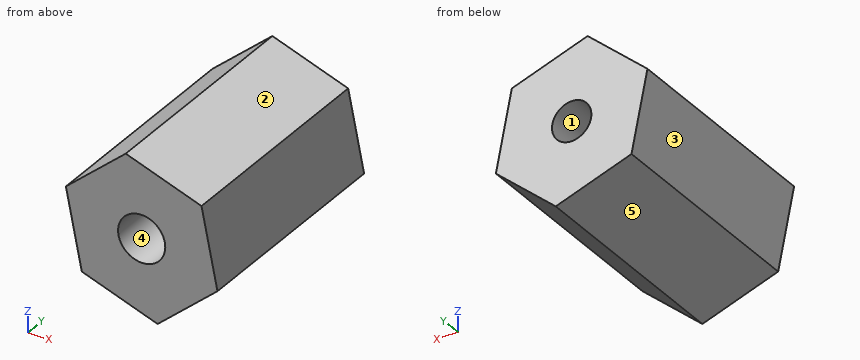
```python
from build123d import *

# Parameters (mm, degrees)
BOSS_EXTRUDE1_DEPTH       = 12.7
F_4_40_TAPPED_HOLE1_D     = 2.2606
F_4_40_TAPPED_HOLE1_DEPTH = 3.571875
F_4_40_TAPPED_HOLE1_TIP   = 0.679152758
F_6_32_TAPPED_HOLE1_D     = 2.7051
F_6_32_TAPPED_HOLE1_DEPTH = 3.556
F_6_32_TAPPED_HOLE1_TIP   = 0.81269403


with BuildPart() as part:
    # Sketch1 → Boss-Extrude1 (new body)
    with BuildSketch(Plane(origin=(0, 0, 0), x_dir=(1, 0, 0), z_dir=(0, 1, 0))):
        Polygon((3.431522356, -3.037425951), (4.346249213, 1.453072558), (0.914726858, 4.490498509), (-3.431522356, 3.037425951), (-4.346249213, -1.453072558), (-0.914726858, -4.490498509), align=None)
    extrude(amount=BOSS_EXTRUDE1_DEPTH)

    # #4-40 Tapped Hole1
    with Locations(Plane(origin=(0, 12.7, 0), x_dir=(1, 0, 0), z_dir=(0, 1, 0))):
        with Locations((0, 0)):
            Hole(F_4_40_TAPPED_HOLE1_D / 2, depth=F_4_40_TAPPED_HOLE1_DEPTH)
            with Locations((0, 0, -(F_4_40_TAPPED_HOLE1_DEPTH + F_4_40_TAPPED_HOLE1_TIP / 2))):  # 118° drill point
                Cone(0, F_4_40_TAPPED_HOLE1_D / 2, F_4_40_TAPPED_HOLE1_TIP, mode=Mode.SUBTRACT)

    # #6-32 Tapped Hole1
    with Locations(Plane(origin=(0, 0, 0), x_dir=(-1, 0, 0), z_dir=(0, -1, 0))):
        with Locations((0, 0)):
            Hole(F_6_32_TAPPED_HOLE1_D / 2, depth=F_6_32_TAPPED_HOLE1_DEPTH)
            with Locations((0, 0, -(F_6_32_TAPPED_HOLE1_DEPTH + F_6_32_TAPPED_HOLE1_TIP / 2))):  # 118° drill point
                Cone(0, F_6_32_TAPPED_HOLE1_D / 2, F_6_32_TAPPED_HOLE1_TIP, mode=Mode.SUBTRACT)


solid = part.part
```
Read the model definition and answer for the solid it produces. Units are mm, in the model's axes. Face numbers are marked on the shaded views. A direction names the side the tool comes from. Give positions to 0.01 mm unless a question says otherwise; leave off trailing zeros. Write each loop counter-clockwise with the first axis right and the second up, starting at its lowest first coordinate (ties: lowest second). Pieces come first, ordered by that corner, then holes. Notation, with made-up numbers: M 40,57.25 L 95,57.25 A31 ccw 95,89.25 Z; hole C 6,-23 d8. An arc over 180 degrees is marked long. Put each result on its own line as item: value. Start each with the question number.
1. Consider line 1 along Z through (x, y) = (0, 11.5); line 2 along Z through (x, y) = (0, 2.8); line 3 along Z through (x, y) = (3, 8.25). Determine where each line is inside the solid, lowest interval first.
2. For a pull along Z with two mould halves and no side action, classify the marked faces 1, 2 and 3 as released by +Z, released by -Z, zero draft, split by the parting line, or undercut.
3. The part is cut by section C-C, the plane y = 1.25. Give the vertices of the cut face in (x, z), and give its area (3 significant figures).
4. The part is cut by section B-B, the plane y = 5.5. Give the vertices of the cut face in (x, z).
5. The part is cut by section A-A, the plane y = 9.75. Give the vertices of the cut face in (x, z).
6. Each of these flat-tipped pins is pushed along its axis until it touches: pin 1 Ø2.5 at (x, z) = (0, 0) entering from +Y; pin 2 Ø1 at (x, y) = (1.5, 8.5) entering from +Z; pin 3 Ø3 at (x, y) = (-2.5, 2) entering from -Z; pin 4 Ø2 at (y, z) = (10, 1.5) entering from +X. Where does it stop, or does it pass through?
7. Which of the six approach directions +Z, -Z, +X, -X, +Y, -Y give full straight-line access (tool end or side, diameter ignored) to the marked faces 4 and 5?
8. The part is cut by section D-D, the plane x = -2.5. Give the vertices of the cut face in (y, z), and give its area (3 significant figures).
Final values:
1. line 1: z = -4.18 to -1.13, 1.13 to 4.18
1. line 2: z = -4.18 to -1.35, 1.35 to 4.18
1. line 3: z = -2.64 to 3.18
2. face 1: undercut
2. face 2: released by +Z
2. face 3: released by -Z
3. outline: M -4.35,1.45 L -3.43,-3.04 L 0.91,-4.49 L 4.35,-1.45 L 3.43,3.04 L -0.91,4.49 Z; hole C 0,0 d2.71
3. area: 48.8 mm²
4. outline: M -4.35,1.45 L -3.43,-3.04 L 0.91,-4.49 L 4.35,-1.45 L 3.43,3.04 L -0.91,4.49 Z
5. outline: M -4.35,1.45 L -3.43,-3.04 L 0.91,-4.49 L 4.35,-1.45 L 3.43,3.04 L -0.91,4.49 Z; hole C 0,0 d2.26
6. pin 1: stops at y = 12.7
6. pin 2: stops at z = 3.85
6. pin 3: stops at z = -3.85
6. pin 4: stops at x = 3.95
7. face 4: -Y
7. face 5: -Z, -X, +Y, -Y
8. outline: M 0,-3.35 L 12.7,-3.35 L 12.7,3.09 L 0,3.09 Z
8. area: 81.7 mm²
